Here's how the part is built. I have some questions about the finished solid (model axes, mm). A direction names the side the tool comes from. Give positions to 0.01 mm unless a question says otherwise; leave off trailing zeros. Order: outer loops, then holes, each group sorted by start corner. A loop starts at its lowest first (then second) coordinate and runs counter-clockwise, first axis right, second up. Notation, with made-up numbers: (68, 70.25) - (93, 70.25) arc R28 cw to (93, 90.25) - close; hole circle Ø4 at (84.25, 36.5). An arc over 180 degrees is marked (long way). One line per question, with ' | ' between items.
from build123d import *

# Parameters (mm, degrees)
CROQUIS1_R              = 19
SALIENTE_EXTRUIR1_DEPTH = 23
CROQUIS2_R              = 17.2
CORTAR_EXTRUIR1_DEPTH   = 10
CROQUIS3_R              = 11.5
CROQUIS3_R_2            = 9.7
SALIENTE_EXTRUIR2_DEPTH = 20
CORTAR_EXTRUIR3_START   = -10
CROQUIS4_R              = 17.2
CORTAR_EXTRUIR3_DEPTH   = 10
SALIENTE_EXTRUIR3_START = 10
CROQUIS5_R              = 11.5
CROQUIS5_R_2            = 9.7
SALIENTE_EXTRUIR3_DEPTH = 10
SALIENTE_EXTRUIR4_DEPTH = 5.5
SALIENTE_EXTRUIR5_START = -2.4
SALIENTE_EXTRUIR5_DEPTH = 2.4
CROQUIS8_R              = 1.5
CORTAR_EXTRUIR4_DEPTH   = 63.451981554


with BuildPart() as part:
    # Croquis1 → Saliente-Extruir1 (new body)
    with BuildSketch(Plane.XY):
        Circle(CROQUIS1_R)
    extrude(amount=SALIENTE_EXTRUIR1_DEPTH)

    # Croquis2 → Cortar-Extruir1 (cut)
    with BuildSketch(Plane.XY.offset(23)):
        Circle(CROQUIS2_R)
    extrude(amount=-CORTAR_EXTRUIR1_DEPTH, mode=Mode.SUBTRACT)

    # Croquis3 → Saliente-Extruir2 (add)
    with BuildSketch(Plane.XY.offset(13)):
        Circle(CROQUIS3_R)
        Circle(CROQUIS3_R_2, mode=Mode.SUBTRACT)
    extrude(amount=SALIENTE_EXTRUIR2_DEPTH)

    # Croquis4 → Cortar-Extruir3 (cut)
    with BuildSketch(Plane(origin=(0, 0, 0), x_dir=(-1, 0, 0), z_dir=(0, 0, -1)).offset(CORTAR_EXTRUIR3_START)):
        with Locations(Location((0, 0, 0), (0, 0, 180))):
            Circle(CROQUIS4_R)
    extrude(amount=CORTAR_EXTRUIR3_DEPTH, mode=Mode.SUBTRACT)

    # Croquis5 → Saliente-Extruir3 (add)
    with BuildSketch(Plane(origin=(0, 0, 10), x_dir=(-1, 0, 0), z_dir=(0, 0, -1)).offset(SALIENTE_EXTRUIR3_START)):
        with Locations(Location((0, 0, 0), (0, 0, 180))):
            Circle(CROQUIS5_R)
        with Locations(Location((0, 0, 0), (0, 0, 180))):
            Circle(CROQUIS5_R_2, mode=Mode.SUBTRACT)
    extrude(amount=-SALIENTE_EXTRUIR3_DEPTH)

    # Croquis6 → Saliente-Extruir4 (add, symmetric)
    with BuildSketch(Plane(origin=(0, 0, 0), x_dir=(0, 0, -1), z_dir=(1, 0, 0))):
        Polygon((-5, 10.008599435), (0, 10.008599435), (0, 10.702416301), (0, 11.5), (0, 49.5), (-5, 49.5), (-5, 11.5), (-5, 10.702416301), align=None)
    extrude(amount=SALIENTE_EXTRUIR4_DEPTH, both=True)

    # Croquis7 → Saliente-Extruir5 (add)
    with BuildSketch(Plane(origin=(0, 0, 0), x_dir=(-1, 0, 0), z_dir=(0, 0, -1)).offset(SALIENTE_EXTRUIR5_START)):
        with BuildLine():
            Line((-13.053420517, -11.200366637), (-5.966841039, -4.144844594))
            Line((-5.966841039, -4.144844594), (-6.870906384, -2.360841833))
            Line((-6.870906384, -2.360841833), (-16.751201418, -3.903492163))
            ThreePointArc((-16.751201418, -3.903492163), (-15.342423747, -7.774961965), (-13.053420517, -11.200366637))
        make_face()
    extrude(amount=SALIENTE_EXTRUIR5_DEPTH)

    # Croquis8 → Cortar-Extruir4 (cut, through all)
    with BuildSketch(Plane(origin=(0, 0, 0), x_dir=(-1, 0, 0), z_dir=(0, 0, -1))):
        with Locations((0, 45.5)):
            Circle(CROQUIS8_R)
    extrude(amount=-CORTAR_EXTRUIR4_DEPTH, mode=Mode.SUBTRACT)


solid = part.part
1) I want a section at A-A (x = 0). State how many separate pieces and enclosed holes the cut face has, plus the area to 3 significant figures.
Model answer:
separate pieces: 2 | enclosed holes: 1 | area: 460 mm2
2) I want a section at C-C (y = 45.5). List the corners of the cut face in (x, z) for me, plus the area to 3 significant figures.
Model answer:
outline: (-5.5, 0) - (-1.5, 0) - (-1.5, 5) - (-5.5, 5) - close; (1.5, 0) - (5.5, 0) - (5.5, 5) - (1.5, 5) - close | area: 40.0 mm2
3) I want a section at B-B (z = 21). List the corners of the cut face in (x, y) for me, plus the area to 3 significant figures.
Model answer:
outline: circle Ø38 at (0, 0); circle Ø23 at (0, 0); hole circle Ø34.4 at (0, 0); hole circle Ø19.4 at (0, 0) | area: 325 mm2
4) On a 3-axis mill with a long thin cutter (end or side, diameter ignored), from which of +Z, -Z, +X, -X, +Y, -Y can I reach the whole of each face in a straight line? I mean faces 1 (the face through (8.07, -2.55, 1.22)), 2 (the face through (0, 14, 5)), 3 (the face through (-17.183, 0.756, 18.07)). Say none if no direction works.
Model answer:
face 1: -Z | face 2: none | face 3: +Z
5) I want a section at D-D (y = 0). List the corners of the cut face in (x, z) for me.
Model answer:
outline: (-19, 0) - (-17.2, 0) - (-17.2, 10) - (-11.5, 10) - (-11.5, 0) - (-9.7, 0) - (-9.7, 10) - (9.7, 10) - (9.7, 0) - (11.5, 0) - (11.5, 10) - (17.2, 10) - (17.2, 0) - (19, 0) - (19, 23) - (17.2, 23) - (17.2, 13) - (11.5, 13) - (11.5, 33) - (9.7, 33) - (9.7, 13) - (-9.7, 13) - (-9.7, 33) - (-11.5, 33) - (-11.5, 13) - (-17.2, 13) - (-17.2, 23) - (-19, 23) - close
6) I'm going to push flat-ended pins straight in: P1, Ø1, axis at x = 5.5, y = 39, coming from the +Z side; P2, Ø11.5, axis at x = 3.5, y = -1, coming from the +Z side; P3, Ø5.5, axis at y = 36.5, z = 1.5, coming from the +X side. Where does each tip first touch, or does it pass through?
Model answer:
P1: stops at z = 5 | P2: stops at z = 13 | P3: stops at x = 5.5
7) Thinking about a two-plate mould opening in Y: for faces 4 (the face through (0, 49.5, 2)), 5 (the face through (0, 34, 5)), 6 (the face through (9.252, 2.914, 22.86)), which applies, +Y half, -Y half, draft (parallel to the pull), parting line (faces both ways), or undercut?
Model answer:
face 4: +Y half | face 5: draft | face 6: undercut
8) Please list where these lines run through material, in increasing order: L1, parallel to Y at x = 0, z = 3; L2, parallel to Y at x = 0, z = 17; L3, parallel to X at y = -1, z = 17.
Model answer:
L1: y = -19 to -17.2, -11.5 to -9.7, 9.7 to 44, 47 to 49.5 | L2: y = -19 to -17.2, -11.5 to -9.7, 9.7 to 11.5, 17.2 to 19 | L3: x = -18.97 to -17.17, -11.46 to -9.65, 9.65 to 11.46, 17.17 to 18.97
